For this review, take the finished solid that the model builds, in its own axes (mm). Face numbers are marked on the shaded views. A direction names the side the tool comes from. Round coordinates to 2 decimals unless told otherwise and drop trailing zeros. Order: outer loops, then holes, each group sorted by start corner. A loop starts at its lowest first (then second) coordinate and runs counter-clockwise, first axis right, second up. Notation, with made-up numbers: (-28.75, -26.5) - (0.25, -26.5) arc R17 ccw to (0.25, 4.5) - close; hole circle Ø3 at (22, 66). An arc over 180 degrees is marked (long way). One line per item, written item: value.
Autodesk Fusion 360 part; units mm, degrees
sketch "Sketch1" plane through (0, 0, 0) normal (0, 1, 0) x (1, 0, 0)
  line L0 (-20.9, 20.9) -> (20.9, 20.9)
  line L1 (20.9, 20.9) -> (20.9, -20.9)
  line L2 (20.9, -20.9) -> (-20.9, -20.9)
  line L3 (-20.9, -20.9) -> (-20.9, 20.9)
  line L4 (-20.9, 20.9) -> (20.9, -20.9) construction
  line L5 (20.9, 20.9) -> (-20.9, -20.9) construction
  line L6 (-20.9, 20.9) -> (-20.9, 16)
  line L7 (-20.9, 16) -> (-16, 16)
  circle A0 centre (-16, 16) radius 2
  circle A1 centre (-16, -16) radius 2
  circle A2 centre (16, -16) radius 2
  circle A3 centre (16, 16) radius 2
  line L8 (-25, 25) -> (25, 25)
  line L9 (25, 25) -> (25, -25)
  line L10 (25, -25) -> (-25, -25)
  line L11 (-25, -25) -> (-25, 25)
  line L12 (-25, 25) -> (25, -25) construction
  line L13 (25, 25) -> (-25, -25) construction
  line L14 (-20.9, 25) -> (-20.9, -25)
  line L15 (20.9, -25) -> (20.9, 25)
  circle A4 centre (0, 0) radius 11.4
  dimension "d1" = 41.8
  dimension "d2" = 41.8
  dimension "d3" = 4.9
  dimension "d4" = 4.9
  dimension "d5" = 4
  dimension "d7" = 360
  dimension "d8" = 50
  dimension "d9" = 50
  dimension "d10" = 22.8
extrude "Extrude1" add sketch "Sketch1" along normal blind 4
extrude "Extrude2" add sketch "Sketch1" against normal blind 39.1 contours L3 L6 L8 L10 L11 L14 | L1 L8 L9 L10 L15
sketch "Sketch2" plane through (-25, 0, 0) normal (-1, 0, 0) x (0, 0, 1)
  line L0 (25, -39.1) -> (25, 4)
  line L1 (25, 4) -> (-25, 4)
  line L2 (-25, 4) -> (-25, -39.1)
  line L3 (-25, -39.1) -> (25, -39.1)
  line L4 (0, -39.1) -> (-10, -39.1)
  line L5 (-10, -39.1) -> (10, -39.1)
  line L6 (10, -39.1) -> (10, -34.1)
  line L7 (10, -34.1) -> (-10, -34.1)
  line L8 (-10, -34.1) -> (-10, -39.1)
  dimension "d15" = 10
  dimension "d16" = 20
  dimension "d17" = 5
sketch "Sketch3" plane through (25, 0, 0) normal (1, 0, 0) x (0, 0, -1)
  line L0 (25, -39.1) -> (25, 4)
  line L1 (25, 4) -> (-25, 4)
  line L2 (-25, 4) -> (-25, -39.1)
  line L3 (-25, -39.1) -> (25, -39.1)
  line L4 (0, -39.1) -> (-10, -39.1)
  line L5 (-10, -39.1) -> (10, -39.1)
  line L6 (10, -39.1) -> (10, -34.1)
  line L7 (10, -34.1) -> (-10, -34.1)
  line L8 (-10, -34.1) -> (-10, -39.1)
  dimension "d18" = 20
  dimension "d19" = 5
extrude "Extrude3" add sketch "Sketch3" along normal blind 15 contours L3 L4 L5 L6 L7 L8
extrude "Extrude4" add sketch "Sketch2" along normal blind 15 contours L3 L4 L5 L6 L7 L8
sketch "Sketch4" plane through (0, -34.1, 0) normal (0, 1, 0) x (-1, 0, 0)
  line L0 (25, 10) -> (25, -10)
  line L1 (25, -10) -> (40, -10)
  line L2 (40, -10) -> (40, 10)
  line L3 (40, 10) -> (25, 10)
  line L4 (40, 0) -> (33, 0)
  circle A0 centre (33, 0) radius 2.8
  dimension "d24" = 7
  dimension "d25" = 5.6
sketch "Sketch5" plane through (0, -34.1, 0) normal (0, 1, 0) x (-1, 0, 0)
  line L0 (-25, -10) -> (-25, 10)
  line L1 (-25, 10) -> (-40, 10)
  line L2 (-40, 10) -> (-40, -10)
  line L3 (-40, -10) -> (-25, -10)
  line L4 (-40, 0) -> (-33, 0)
  circle A0 centre (-33, 0) radius 2.8
  dimension "d26" = 7
  dimension "d27" = 5.6
extrude "Extrude5" cut sketch "Sketch4" sketch "Sketch5" against normal blind 30 contours A0 of sketch 2 contours A0
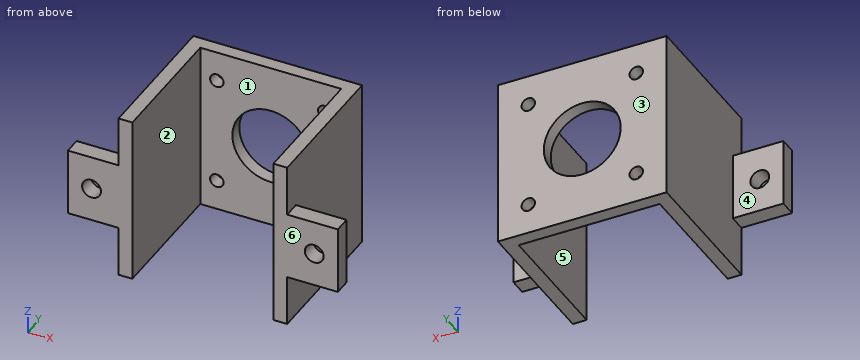
Item 1: Take a section at C-C (x = -16). Write out the cut boundary in (y, z).
Returned:
outline: (0, -25) - (4, -25) - (4, -18) - (0, -18) - close; (0, -14) - (4, -14) - (4, 14) - (0, 14) - close; (0, 18) - (4, 18) - (4, 25) - (0, 25) - close
Item 2: For P1, Ø1.5, axis at x = 33, y = -36.5, coming from the -Z side; P2, Ø5, axis at y = -16, z = 12, coming from the -X side; P3, Ø6.5, axis at x = 16, z = 16, coming from the -Y side; P4, Ø16.5, axis at x = -31, z = 4, coming from the +Y side, all flat-tipped, find the tip position at first contact; note any pin that passes through.
Returned:
P1: z = -10
P2: x = -25
P3: y = 0
P4: y = 4
Item 3: Machinability: for the marked faces 4, 5 and 6, which of the approach directions +Z, -Z, +X, -X, +Y, -Y give a long, thin tool a straight path to every point of the face, cutting with its end or side? Answer none if there is none.
Returned:
face 4: +Z, -Z, -X, +Y
face 5: +Z, -Z, -Y
face 6: +Z, -Z, +X, -X, -Y
Item 4: The part is to be moulded in two halves that separate along X. For the marked faces 1, 2 and 3, say which applies: +X half, -X half, draft (parallel to the pull), parting line (faces both ways), or undercut.
Returned:
face 1: undercut
face 2: undercut
face 3: draft
Item 5: Wall thickness on line 1 (Z direction, x = 16, y = 2.55); line 2 (Z direction, x = 0, y = 3.15): over which ranges is each line inside the solid? List them lowest first.
Returned:
line 1: -25 to -18, -14 to 14, 18 to 25
line 2: -25 to -11.4, 11.4 to 25
Item 6: Take a section at B-B (y = -7). Write out the cut boundary in (x, z).
Returned:
outline: (-25, -25) - (-20.9, -25) - (-20.9, 25) - (-25, 25) - close; (20.9, -25) - (25, -25) - (25, 25) - (20.9, 25) - close
Item 7: Take a section at D-D (z = 0). Write out the cut boundary in (x, y).
Returned:
outline: (-40, -39.1) - (-35.8, -39.1) - (-35.8, -34.1) - (-40, -34.1) - close; (-30.2, -39.1) - (-20.9, -39.1) - (-20.9, 0) - (-11.4, 0) - (-11.4, 4) - (-25, 4) - (-25, -34.1) - (-30.2, -34.1) - close; (11.4, 0) - (20.9, 0) - (20.9, -39.1) - (30.2, -39.1) - (30.2, -34.1) - (25, -34.1) - (25, 4) - (11.4, 4) - close; (35.8, -39.1) - (40, -39.1) - (40, -34.1) - (35.8, -34.1) - close
Item 8: Take a section at A-A (x = 0). Write out the cut boundary in (y, z), plus the area to 3 significant figures.
Returned:
outline: (0, -25) - (4, -25) - (4, -11.4) - (0, -11.4) - close; (0, 11.4) - (4, 11.4) - (4, 25) - (0, 25) - close
area: 109 mm^2
